Source: CAD feature listing. Evaluate the final solid. Frame: model axes, mm. A direction names the side the tool comes from. Coordinates: 2 decimals unless noted, no trailing zeros. Loops run counter-clockwise (first coordinate to the right, second up) from the corner with the lowest first, then second, coordinate; pieces in that order, holes last.
```python
from build123d import *

# Parameters (mm, degrees)
SKETCH1_W           = 180
SKETCH1_H           = 30
BOSS_EXTRUDE1_DEPTH = 8
SKETCH3_W           = 16
SKETCH3_H           = 15
CUT_EXTRUDE1_DEPTH  = 8


with BuildPart() as part:
    # Sketch1 → Boss-Extrude1 (new body)
    with BuildSketch(Plane(origin=(0, 0, 0), x_dir=(1, 0, 0), z_dir=(0, 1, 0))):
        Rectangle(SKETCH1_W, SKETCH1_H)
    extrude(amount=BOSS_EXTRUDE1_DEPTH)

    # Sketch3 → Cut-Extrude1 (cut)
    with BuildSketch(Plane(origin=(0, 8, 0), x_dir=(1, 0, 0), z_dir=(0, 1, 0))):
        with Locations((-72, -7.5)):
            Rectangle(SKETCH3_W, SKETCH3_H)
    cut_extrude1 = extrude(amount=-CUT_EXTRUDE1_DEPTH, mode=Mode.SUBTRACT)

    # Mirror1: Cut-Extrude1 across plane
    add(cut_extrude1.mirror(Plane(origin=(0, 0, 0), x_dir=(0, 0, 1), z_dir=(1, 0, 0))), mode=Mode.SUBTRACT)


solid = part.part
```
Q1. Section query A-A on z = 10. Return the cut outline in (x, y), then the cut area to 3 significant figures.
Q2. Draft query along X for faces 1 (the flat face through (-1, 4, 15)), 2 (the flat face through (-72, 4, 0)), 3 (the flat face through (90, 4, 0)). Return one class per face: released by +X, released by -X, zero draft, split by the parting line, or undercut.
Q3. Reachability of faces 4 (the flat face through (-80, 4, 8)), 5 (the flat face through (-1, 8, 0)) from +Z, -Z, +X, -X, +Y, -Y: full face, straight path, thin tool, end or side. Return the list, or none.
Q4. First-contact query: pin 1 Ø6 at (x, z) = (-40.5, 5.5) entering from -Y. Flat tip, straight axial feed; report the tip coordinate or a pass-through.
Q5. Section query B-B on y = 5.5. Return the cut outline in (x, z), then the cut area to 3 significant figures.
Q6. Material intervals for line 1 along X through (y, z) = (4.5, 5); line 2 along Z through (x, y) = (-69.5, 7), sorted ascending.
Resolved:
1. outline: (-90, 0) - (-80, 0) - (-80, 8) - (-90, 8) - close; (-64, 0) - (64, 0) - (64, 8) - (-64, 8) - close; (80, 0) - (90, 0) - (90, 8) - (80, 8) - close
1. area: 1,180 mm2
2. face 1: zero draft
2. face 2: undercut
2. face 3: released by +X
3. face 4: +Z, +Y, -Y
3. face 5: +Z, -Z, +X, -X, +Y
4. pin 1: stops at y = 0
5. outline: (-90, -15) - (90, -15) - (90, 15) - (80, 15) - (80, 0) - (64, 0) - (64, 15) - (-64, 15) - (-64, 0) - (-80, 0) - (-80, 15) - (-90, 15) - close
5. area: 4,920 mm2
6. line 1: x = -90 to -80, -64 to 64, 80 to 90
6. line 2: z = -15 to 0
